Verification items for this drawing (mm, ordinates from the low corner). A direction names the side the tool comes from. Round coordinates to 2 decimals unless told otherwise and drop trailing zeros. Order: outer loops, then holes, each group sorted by start corner. A loop starts at its lowest first (then second) coordinate and runs counter-clockwise, first axis right, second up.
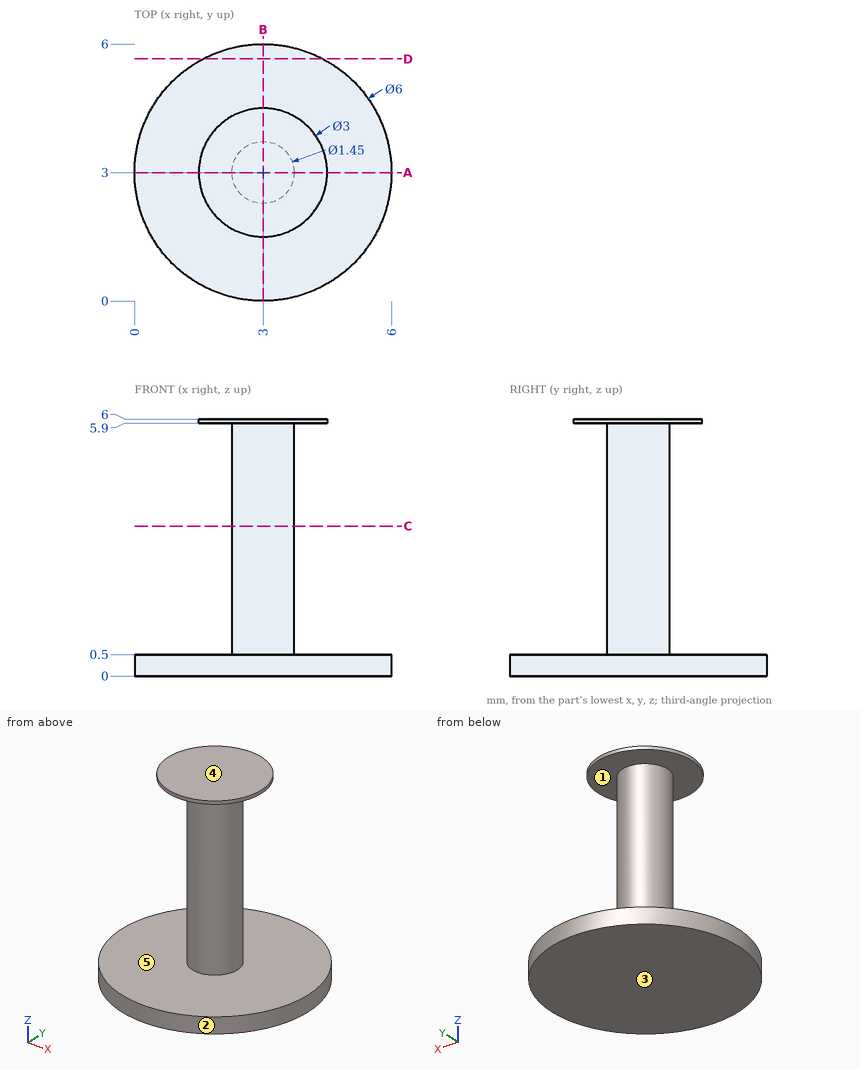
Item 1: Scan lines: line 1 along Z through (x, y) = (3.4, 5.6); line 2 along X through (y, z) = (3.25, 2.6); line 3 along Y through (x, z) = (3.45, 1.05). Record each from-to range of solid material in increasing order.
Answer:
line 1: z = 0 to 0.5
line 2: x = 2.32 to 3.68
line 3: y = 2.43 to 3.57
Item 2: Sectioned sample at C-C (z = 3.5). Record the cut outline in (x, y) (3 decimals).
Answer:
outline: circle Ø1.45 at (3, 3)
Item 3: Sectioned sample at A-A (y = 3). Record the cut outline in (x, z) (3 decimals), and give its area (3 significant figures).
Answer:
outline: (0, 0) - (6, 0) - (6, 0.5) - (3.725, 0.5) - (3.725, 5.9) - (4.5, 5.9) - (4.5, 6) - (1.5, 6) - (1.5, 5.9) - (2.275, 5.9) - (2.275, 0.5) - (0, 0.5) - close
area: 11.1 mm2
Item 4: Release check for a two-part mould opening along Z. For the marked faces 3, 4 and 5 record: released by +Z, released by -Z, zero draft, split by the parting line, or undercut.
Answer:
face 3: released by -Z
face 4: released by +Z
face 5: undercut
Item 5: Sectioned sample at D-D (y = 5.65). Record the cut outline in (x, z), and give its area (3 significant figures).
Answer:
outline: (1.59, 0) - (4.41, 0) - (4.41, 0.5) - (1.59, 0.5) - close
area: 1.41 mm2
Item 6: Go/stop test with flat-tipped pins: P1, Ø3, axis at x = 1.5, z = 1, coming from the +Y side; P2, Ø1.5, axis at x = 2.5, z = 5.5, coming from the -Y side; P3, Ø1, axis at x = 2, z = 3.5, coming from the -Y side (3 decimals). Record where each tip stops, or that it passes through.
Answer:
P1: stops at y = 6
P2: stops at y = 1.5
P3: stops at y = 2.475
Item 7: Access from +Z, -Z, +X, -X, +Y, -Y to the whole of each face (thin tool, end or side, straight path). Record for the marked faces 1 and 2.
Answer:
face 1: none
face 2: +Z, -Z
